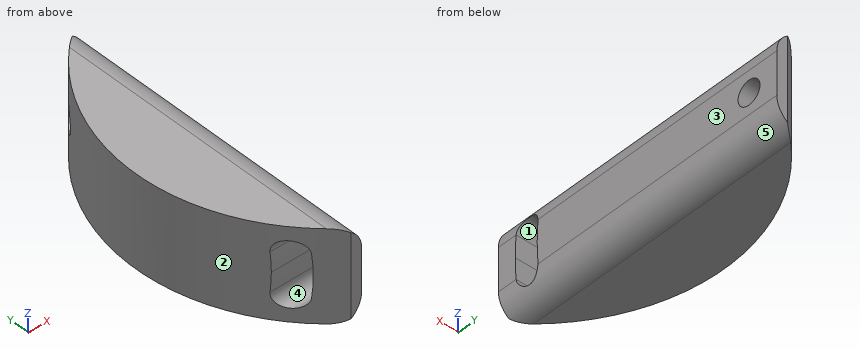
from build123d import *

# Parameters (mm, degrees)
F1_DEPTH    = 19.05
F3_DEPTH    = 25.4
F4_D        = 5
F4_DEPTH    = 15.6972
F4_TIP      = 1.5021515476
F5_T1_DEPTH = 88.9


# Not quite as in the source:
# - a fillet or chamfer that OpenCascade refuses, or shapes differently, is made with other operations: its cross-section is extruded or revolved along the edge and cut away or added


with BuildPart() as f1:
    # F0 (on Top) → F1 (new body)
    with BuildSketch(Plane.XY):
        with BuildLine():
            Line((-22.0673531294, 31.75), (-24.2402065279, 31.75))
            ThreePointArc((-24.2402065279, 31.75), (-39.9455894, 0), (-24.2402065279, -31.75))
            Line((-24.2402065279, -31.75), (-22.0673531294, -31.75))
            Line((-22.0673531294, -31.75), (-22.0673531294, 31.75))
        make_face()
    extrude(amount=F1_DEPTH)

    # F2 (on face) → F3 (cut)
    with BuildSketch(Plane.YZ.offset(-22.0673531294)):
        with BuildLine():
            ThreePointArc((-27.7153407028, 13.9654662391), (-27.8542875294, 11.747165191), (-27.90063, 9.525))
            Line((-27.90063, 9.525), (-22.89937, 9.525))
            ThreePointArc((-22.89937, 9.525), (-22.8573758972, 11.538656851), (-22.7314666127, 13.5488121361))
            ThreePointArc((-22.7314666127, 13.5488121361), (-25.0150766063, 16.2490762326), (-27.7153407028, 13.9654662391))
        make_face()
        with BuildLine():
            Line((-22.89937, 9.525), (-27.90063, 9.525))
            ThreePointArc((-27.90063, 9.525), (-27.8542875294, 7.302834809), (-27.7153407028, 5.0845337609))
            ThreePointArc((-27.7153407028, 5.0845337609), (-25.0150766063, 2.8009237674), (-22.7314666127, 5.5011878639))
            ThreePointArc((-22.7314666127, 5.5011878639), (-22.8573758972, 7.511343149), (-22.89937, 9.525))
        make_face()
    extrude(amount=-F3_DEPTH, mode=Mode.SUBTRACT)

    # F4
    with Locations(Plane.YZ.offset(-22.0673531294)):
        with Locations((25.4, 9.525)):
            Hole(F4_D / 2, depth=F4_DEPTH)
            with Locations((0, 0, -(F4_DEPTH + F4_TIP / 2))):  # 118° drill point
                Cone(0, F4_D / 2, F4_TIP, mode=Mode.SUBTRACT)

    # F5: fillet of radius 5.08 on 2 edges, made by hand

    # F5_s2 → F5_t1 (cut)
    with BuildSketch(Plane.XZ.offset(-44.45)):
        with BuildLine():
            ThreePointArc((-22.0673531294, 13.97), (-23.555250681, 17.5621024484), (-27.1473531294, 19.05))
            Line((-27.1473531294, 19.05), (-22.0673531294, 19.05))
            Line((-22.0673531294, 19.05), (-22.0673531294, 13.97))
        make_face()
        with BuildLine():
            ThreePointArc((-22.0673531294, 5.08), (-23.555250681, 1.4878975516), (-27.1473531294, 0))
            Line((-27.1473531294, 0), (-22.0673531294, 0))
            Line((-22.0673531294, 0), (-22.0673531294, 5.08))
        make_face()
    extrude(amount=F5_T1_DEPTH, mode=Mode.SUBTRACT)


solid = f1.part
Source: CAD feature listing. Evaluate the final solid. Frame: model axes, mm. Face numbers are marked on the shaded views. A direction names the side the tool comes from. Give positions to 0.01 mm unless a question says otherwise; leave off trailing zeros. Order: outer loops, then holes, each group sorted by start corner. A loop starts at its lowest first (then second) coordinate and runs counter-clockwise, first axis right, second up. Notation, with made-up numbers: (22.5, 20.25) -> (36.5, 20.25) arc R22 ccw to (36.5, 45.25) -> close; hole circle Ø2 at (50.5, 8.5). An arc over 180 degrees is marked (long way). Use a Markdown table: item, result.
1) Contact query for flat-ended pins moving along their axis: P1, Ø6, axis at x = -29.5, z = 9.5, coming from the +Y side; P2, Ø8, axis at x = -25.5, y = -6.5, coming from the +Z side; P3, Ø5, axis at x = -36.5, z = 9, coming from the -Y side; P4, Ø4, axis at x = -35.5, z = 14.5, coming from the +Y side. Output: stop coordinate, or through.
Answer list:
| item | result |
|---|---|
| P1 | y = 29.89 |
| P2 | z = 19.05 |
| P3 | y = -20.97 |
| P4 | y = 21.76 |
2) Section query C-C, the plane y = 25.4. Return the cut outline in (x, z) (3 decimals).
Answer list:
| item | result |
|---|---|
| outline | (-30.83, 0) -> (-27.147, 0) arc R5.08 ccw to (-22.067, 5.08) -> (-22.067, 7.025) -> (-30.83, 7.025) -> close; (-30.83, 12.025) -> (-22.067, 12.025) -> (-22.067, 13.97) arc R5.08 ccw to (-27.147, 19.05) -> (-30.83, 19.05) -> close |
3) Reachability of the marked faces 4 and 5 from +Z, -Z, +X, -X, +Y, -Y: full face, straight path, thin tool, end or side. Return the list, or none.
Answer list:
| item | result |
|---|---|
| face 4 | +X, -X |
| face 5 | -Z, +X, +Y, -Y |
4) Mould query, pull axis Y, two halves, no side actions, for the marked faces 1, 2 and 3. Classes: +Y half, -Y half, draft (parallel to the pull), parting line (faces both ways), or undercut.
Answer list:
| item | result |
|---|---|
| face 1 | undercut |
| face 2 | parting line |
| face 3 | draft |
5) Section query A-A, the plane z = 4.25. Return the cut outline in (x, y), then the cut area to 3 significant figures.
Answer list:
| item | result |
|---|---|
| outline | (-32.69, -22.95) -> (-22.14, -22.95) -> (-22.14, 31.75) -> (-24.24, 31.75) arc R39.95 ccw to start; (-28.98, -27.5) arc R39.95 ccw to (-24.24, -31.75) -> (-22.14, -31.75) -> (-22.14, -27.5) -> close |
| area | 790 mm² |
6) Section query D-D, the plane x = -31.25. Return the cut outline in (y, z) (3 decimals).
Answer list:
| item | result |
|---|---|
| outline | (-24.881, 0) -> (24.881, 0) -> (24.881, 7.079) arc R2.5 cw to (24.881, 11.971) -> (24.881, 19.05) -> (-24.881, 19.05) -> (-24.881, 16.234) arc R2.501 cw to (-22.731, 13.549) arc R48.299 ccw to (-22.731, 5.501) arc R2.501 cw to (-24.881, 2.816) -> close |
7) Ray query, line 1 along Z through (x, y) = (-29.25, 25.4) (3 decimals); line 2 along Z through (x, y) = (-27.25, -25.5); line 3 along Y through (x, z) = (-34, 4.25). Return the intervals inside material, ascending. Write a range as [from, to].
Answer list:
| item | result |
|---|---|
| line 1 | [0, 7.025], [12.025, 19.05] |
| line 2 | [0, 2.81], [16.24, 19.05] |
| line 3 | [-20.97, 20.97] |
8) Section query B-B, the plane x = -26.25. Return the cut outline in (y, z) (3 decimals), then the cut area to 3 significant figures.
Answer list:
| item | result |
|---|---|
| outline | (-30.11, 0.08) -> (30.11, 0.08) -> (30.11, 18.97) -> (-30.11, 18.97) -> close; hole (-27.715, 5.085) arc R2.501 ccw to (-22.731, 5.501) arc R48.299 cw to (-22.731, 13.549) arc R2.501 ccw to (-27.715, 13.965) arc R53.301 ccw to start; hole circle Ø5 at (25.4, 9.525) |
| area | 1,060 mm² |
